CAD build for the part. Positions are in the model's coordinates, mm. Face numbers are marked on the shaded views. Coordinates: 2 decimals unless noted, no trailing zeros. Loops run counter-clockwise (first coordinate to the right, second up) from the corner with the lowest first, then second, coordinate; pieces in that order, holes last. Notation, with made-up numbers: (-34.5, 71.5) -> (-21.5, 71.5) arc R33 cw to (-21.5, 101.5) -> close; hole circle Ø2 at (-25, 30). An arc over 180 degrees is marked (long way). Return JSON: item names as keys, results as strings. Group by question number.
(1) Probe L1, parallel to X at y = 54, z = 0.5; L2, parallel to Z at x = -9, y = 83.5. List the from-to ranges inside material, lowest first.
(2) Mould opens along X. For the marked faces 1, 2 and 3 say: pulls with the +X half, pulls with the -X half, needs draft (parallel to the pull), parting line crosses it, or undercut.
(3) Flat gauge pins, fed straight in: pin 1 Ø9.5 at (x, y) = (0, 12) entering from -Z; pin 2 Ø2 at (x, z) = (28.5, -21.5) entering from +Y; pin 3 Ø3 at (y, z) = (28, -25) entering from +X. Where does each tip first touch, or does it go through?
(4) Saw through at A-A on y = 80. Write the cut outline in (x, z).
(5) Saw through at B-B on y = 12. Write the cut outline in (x, z), then the cut area to 3 significant figures.
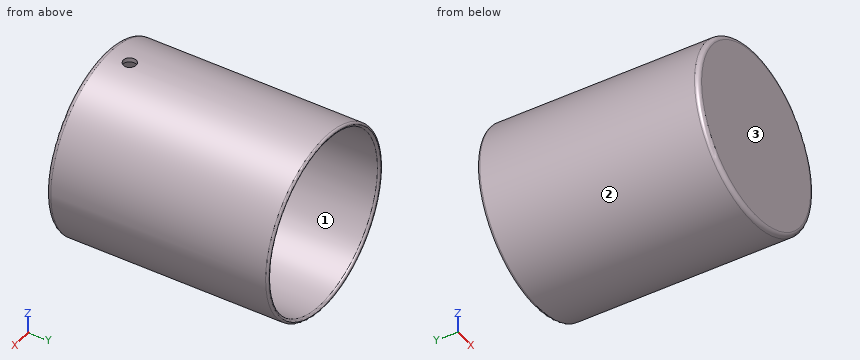
Autodesk Inventor part; units mm, degrees
ref_plane "YZ Plane" through (0, 0, 0) normal (1, 0, 0) x (0, 1, 0)
ref_plane "XZ Plane" through (0, 0, 0) normal (0, 1, 0) x (-1, 0, 0)
ref_plane "XY Plane" through (0, 0, 0) normal (0, 0, 1) x (1, 0, 0)
sketch "Sketch1" plane through (0, 0, 0) normal (0, 1, 0) x (-1, 0, 0)
  circle A0 centre (0, 0) radius 42
  dimension "d0" = 84
extrude "Extrusion1" add sketch "Sketch1" along normal blind 2
sketch "Sketch2" plane through (0, 2, 0) normal (0, 1, 0) x (1, 0, 0)
  circle A0 centre (0, 0) radius 42
  circle A1 centre (0, 0) radius 40
  dimension "d3" = 80
  dimension "d6" = 84
extrude "Extrusion2" add sketch "Sketch2" along normal blind 100
fillet "Fillet1" radius 2 1 edges at (42, 0, 0)
fillet "Fillet2" radius 1 2 edges at (-42, 102, 0) (-40, 102, 0)
fillet "Fillet3" radius 1 1 edges at (-40, 2, 0)
sketch "Sketch3" plane through (0, 0, 0) normal (0, 0, 1) x (1, 0, 0)
  line L0 (-42, 2) -> (42, 2)
  line L1 (0, 2) -> (0, 12)
  circle A0 centre (0, 12) radius 3
  point P0 (0, 0)
  dimension "d10" = 10
  dimension "d11" = 6
extrude "Extrusion3" cut sketch "Sketch3" along normal through all
ref_plane "Work Plane1" through (0, 0, 42) normal (0, 0, 1) x (1, 0, 0)
properties part number "Reservoir"
Geometry results:
{
 "1": {"L1": "-42 to -40, 40 to 42", "L2": "-41.02 to -38.97, 38.97 to 41.02"},
 "2": {"face 1": "undercut", "face 2": "parting line crosses it", "face 3": "needs draft"},
 "3": {"pin 1": "z = -42", "pin 2": "y = 2", "pin 3": "x = 34.81"},
 "4": {"outline": "circle Ø84 at (0, 0); hole circle Ø80 at (0, 0)"},
 "5": {"outline": "(-3, 39.89) -> (-3, 41.89) arc R42 ccw (long way) to (3, 41.89) -> (3, 39.89) arc R40 cw (long way) to start", "area": "503 mm²"}
}
